Geometry check sheet. Reference: the model listing, model coordinates, mm. A direction names the side the tool comes from. Give positions to 0.01 mm unless a question says otherwise; leave off trailing zeros. Loops run counter-clockwise (first coordinate to the right, second up) from the corner with the lowest first, then second, coordinate; pieces in that order, holes last.
```python
from build123d import *

# Parameters (mm, degrees)
SKETCH1_R                    = 4.25
BOSS_EXTRUDE1_DEPTH          = 20
CUT_EXTRUDE_THIN1_DEPTH      = 66.294046436
CUT_EXTRUDE_THIN1_DEPTH_BACK = 20
SKETCH3_W                    = 3
SKETCH3_H                    = 60.5
SKETCH4_W                    = 27.75
SKETCH4_H                    = 20
BOSS_EXTRUDE2_DEPTH          = 5
SKETCH5_R                    = 2.75
CUT_EXTRUDE1_DEPTH           = 5
CHAMFER1_SIZE                = 2
CHAMFER2_SIZE                = 2
SKETCH6_R                    = 2.75
CUT_EXTRUDE2_DEPTH           = 35
CUT_EXTRUDE3_DEPTH           = 3
SKETCH8_R                    = 4
CUT_EXTRUDE4_DEPTH           = 4


with BuildPart() as part:
    # Sketch1 → Boss-Extrude1 (new body)
    with BuildSketch(Plane(origin=(0, 0, 0), x_dir=(1, 0, 0), z_dir=(0, 1, 0))):
        with BuildLine():
            Line((-14.25, 0), (-14.25, -60.5))
            Line((-14.25, -60.5), (14.25, -60.5))
            Line((14.25, -60.5), (14.25, 0))
            ThreePointArc((14.25, 0), (0, 14.25), (-14.25, 0))
        make_face()
        with Locations(Location((0, 0, 0), (0, 0, 270))):
            Circle(SKETCH1_R, mode=Mode.SUBTRACT)
    extrude(amount=BOSS_EXTRUDE1_DEPTH)

    # Sketch3 → Cut-Extrude-Thin1 (cut, two sides: drawn at the far end of the back side and taken through both)
    with BuildSketch(Plane(origin=(0, 20, 0), x_dir=(1, 0, 0), z_dir=(0, 1, 0)).offset(-CUT_EXTRUDE_THIN1_DEPTH_BACK)):
        with Locations((0, -30.25)):
            Rectangle(SKETCH3_W, SKETCH3_H)
    extrude(amount=CUT_EXTRUDE_THIN1_DEPTH + CUT_EXTRUDE_THIN1_DEPTH_BACK, mode=Mode.SUBTRACT)

    # Sketch4 → Boss-Extrude2 (add)
    with BuildSketch(Plane.XY.offset(60.5)):
        with Locations((-15.375, 10)):
            Rectangle(SKETCH4_W, SKETCH4_H)
    boss_extrude2 = extrude(amount=-BOSS_EXTRUDE2_DEPTH)

    # Mirror1: Boss-Extrude2 across plane
    add(boss_extrude2.mirror(Plane(origin=(0, 0, 0), x_dir=(0, 0, 1), z_dir=(1, 0, 0))))

    # Sketch5 → Cut-Extrude1 (cut)
    with BuildSketch(Plane(origin=(0, 0, 55.5), x_dir=(-1, 0, 0), z_dir=(0, 0, -1))):
        with Locations((21.75, 10)):
            Circle(SKETCH5_R)
        with BuildLine():
            Line((-24.25, 12.75), (-19.25, 12.75))
            ThreePointArc((-19.25, 12.75), (-16.5, 10), (-19.25, 7.25))
            Line((-19.25, 7.25), (-24.25, 7.25))
            ThreePointArc((-24.25, 7.25), (-27, 10), (-24.25, 12.75))
        make_face()
    extrude(amount=-CUT_EXTRUDE1_DEPTH, mode=Mode.SUBTRACT)

    # Chamfer1
    chamfer1_edges = [part.edges().sort_by_distance(p)[0] for p in [
        (-14.25, 10, 55.5),
        (14.25, 10, 55.5),
    ]]
    chamfer(chamfer1_edges, length=CHAMFER1_SIZE)

    # Chamfer2
    chamfer2_edges = [part.edges().sort_by_distance(p)[0] for p in [
        (-29.25, 20, 58),
        (-29.25, 0, 58),
        (29.25, 0, 58),
        (29.25, 20, 58),
    ]]
    chamfer(chamfer2_edges, length=CHAMFER2_SIZE)

    # Sketch6 → Cut-Extrude2 (cut)
    with BuildSketch(Plane(origin=(14.25, 0, 0), x_dir=(0, 0, -1), z_dir=(1, 0, 0))):
        with Locations((-26.75, 10)):
            Circle(SKETCH6_R)
    extrude(amount=-CUT_EXTRUDE2_DEPTH, mode=Mode.SUBTRACT)

    # Sketch7 → Cut-Extrude3 (cut)
    with BuildSketch(Plane(origin=(14.25, 0, 0), x_dir=(0, 0, -1), z_dir=(1, 0, 0))):
        Polygon((-22.708548116, 10), (-24.729274058, 13.5), (-28.770725942, 13.5), (-30.791451884, 10), (-28.770725942, 6.5), (-24.729274058, 6.5), align=None)
    extrude(amount=-CUT_EXTRUDE3_DEPTH, mode=Mode.SUBTRACT)

    # Sketch8 → Cut-Extrude4 (cut)
    with BuildSketch(Plane.ZY.offset(14.25)):
        with Locations((26.75, 10)):
            Circle(SKETCH8_R)
    extrude(amount=-CUT_EXTRUDE4_DEPTH, mode=Mode.SUBTRACT)


solid = part.part
```
1) Scan lines: line 1 along Y through (x, z) = (-21.75, 59.2); line 2 along X through (y, z) = (14.75, 49.5); line 3 along Y through (x, z) = (-11.75, 26.75). Record each from-to range of solid material in increasing order.
2) Depth check by flat-ended pin: P1, Ø1, axis at y = 11, z = 40.5, coming from the -X side; P2, Ø3.5, axis at x = 13, z = 26.5, coming from the -Y side; P3, Ø8, axis at x = -23, y = 5.5, coming from the -Z side; P4, Ø10, axis at y = 3.5, z = 2.5, coming from the +X side. Enter the tip coordinate at first touch or a pass-through.
3) Tool access check on faces 1 (the flat face through (11.25, 13, 26)), 2 (the flat face through (-24, 8, 55.5)), 3 (the flat face through (22, 12.75, 58)). Record the directions out of +Z, -Z, +X, -X, +Y, -Y that give a thin tool (end or side, any length) a straight path to the whole face; none if there is none.
4) Mould release check, pull along Y, two halves, no side actions. Record for faces 4 (the flat face through (28.24, 19.01, 58.04)), 5 (the flat face through (1.5, 10, 33)), 6 (the flat face through (-10.25, 7, 26)): +Y half, -Y half, draft (parallel to the pull), parting line (faces both ways), or undercut.
5) Sectioned sample at D-D on y = 3.25. Enter the section's corners in (x, z), plus the area to 3 significant figures.
6) Sectioned sample at C-C on x = -21.75. Enter the section's corners in (y, z).
7) Sectioned sample at B-B on x = 2.5. Enter the section's corners in (y, z), plus the area to 3 significant figures.
8) Sectioned sample at A-A on z = 18.5. Enter the section's corners in (x, y).
Determined:
1. line 1: y = 0 to 7.25, 12.75 to 20
1. line 2: x = -14.25 to -1.5, 1.5 to 14.25
1. line 3: y = 0 to 6, 14 to 20
2. P1: stops at x = -14.25
2. P2: stops at y = 0
2. P3: stops at z = 55.5
2. P4: stops at x = 14.25
3. face 1: +X
3. face 2: -Z, -X, +Y, -Y
3. face 3: +Z, -Z
4. face 4: +Y half
4. face 5: draft
4. face 6: undercut
5. outline: (-29.25, 55.5) - (-16.25, 55.5) - (-14.25, 53.5) - (-14.25, 0) arc R14.25 ccw to (14.25, 0) - (14.25, 53.5) - (16.25, 55.5) - (29.25, 55.5) - (29.25, 60.5) - (1.5, 60.5) - (1.5, 3.98) arc R4.25 cw (long way) to (-1.5, 3.98) - (-1.5, 60.5) - (-29.25, 60.5) - close
5. area: 1,970 mm2
6. outline: (0, 55.5) - (7.25, 55.5) - (7.25, 60.5) - (0, 60.5) - close; (12.75, 55.5) - (20, 55.5) - (20, 60.5) - (12.75, 60.5) - close
7. outline: (0, -14.03) - (20, -14.03) - (20, -3.44) - (0, -3.44) - close; (0, 3.44) - (20, 3.44) - (20, 60.5) - (0, 60.5) - close; hole circle Ø5.5 at (10, 26.75)
7. area: 1,330 mm2
8. outline: (-14.25, 0) - (-1.5, 0) - (-1.5, 20) - (-14.25, 20) - close; (1.5, 0) - (14.25, 0) - (14.25, 20) - (1.5, 20) - close
